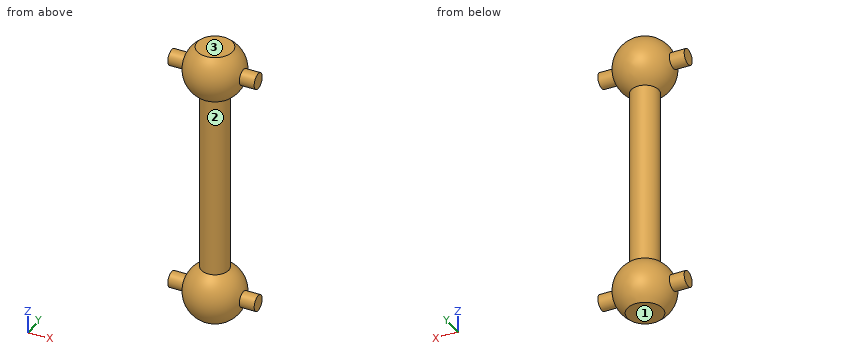
from build123d import *
from build123d.topology import SkipClean

# Parameters (mm, degrees)
SKETCH_1_R      = 3.5
EXTRUDE_1_DEPTH = 25
SKETCH_3_R      = 2
EXTRUDE_2_DEPTH = 11


with BuildPart() as part:
    # Sketch 1 → Extrude 1 (new, symmetric)
    with BuildSketch(Plane.XY):
        Circle(SKETCH_1_R)
    extrude(amount=EXTRUDE_1_DEPTH, both=True)

    # Sketch 2 → Revolve 1 (revolve)
    with SkipClean():  # the faces are left unmerged after this step: merging them gives an invalid solid
        with BuildSketch(Plane(origin=(0, 0, 0), x_dir=(0, 0, -1), z_dir=(1, 0, 0))):
            with BuildLine():
                Line((36, 0), (36, 4.5))
                ThreePointArc((36, 4.5), (27.628291755, 7.115124735), (22.5, 0))
                Line((22.5, 0), (36, 0))
            make_face()
            with BuildLine():
                Line((36, -4.5), (36, 0))
                Line((36, 0), (22.5, 0))
                ThreePointArc((22.5, 0), (27.628291755, -7.115124735), (36, -4.5))
            make_face()
        revolve_1 = revolve(axis=Axis((0, 0, -22.5), (0, 0, -1)))
    add(part.part.scale(1), mode=Mode.REPLACE)  # the faces are merged on a copy

    # Sketch 3 → Extrude 2 (add, symmetric)
    with BuildSketch(Plane(origin=(0, 0, 0), x_dir=(0, 0, -1), z_dir=(1, 0, 0))):
        with Locations(Location((30, 0, 0), (0, 0, 180))):
            Circle(SKETCH_3_R)
    extrude_2 = extrude(amount=EXTRUDE_2_DEPTH, both=True)

    # Mirror 1: Revolve 1, Extrude 2 across plane
    add(revolve_1.mirror(Plane.XY))
    add(extrude_2.mirror(Plane.XY))


solid = part.part
CAD build for the part. Positions are in the model's coordinates, mm. Face numbers are marked on the shaded views. Round coordinates to 2 decimals unless told otherwise and drop trailing zeros. Loops run counter-clockwise (first coordinate to the right, second up) from the corner with the lowest first, then second, coordinate; pieces in that order, holes last.
(1) Cut at B-B (y = 0). Give the cut face in (x, z).
(2) Cut at A-A (x = 0). Give the cut face in (y, z), plus the area to 3 significant figures.
(3) Wall check: line 1 along Y through (x, z) = (-6, -30); line 2 along Z through (x, y) = (-1, -3.5); line 3 along Z through (x, y) = (-5, 1.5). Give the ranges that are in metal, low to high.
(4) Two-plate mould, pull along Z, no slides. Class the marked faces 1, 2 and 3: +Z half, -Z half, draft (parallel to the pull), parting line (faces both ways), or undercut.
(5) Cut at D-D (y = 6.25). Give the cut face in (x, z), plus the area to 3 significant figures.
(6) Cut at C-C (z = -30). Give the cut face in (x, y), plus the area to 3 significant figures.
(7) Drop flat-ended pins along their axis: pin 1 (6 mm diameter, centred on y = -2, z = -15, fed in from +X); pin 2 (1.5 mm diameter, centred on y = 1.5, z = 21.5, fed in from +X); pin 3 (8 mm diameter, centred on y = -5.5, z = -17.5, fed in from +X); pin 4 (6 mm diameter, centred on y = -0.5, z = 27, fed in from -X). Give the stop position or say it passes through.
Findings below:
1. outline: (-11, -32) - (-7.23, -32) arc R7.5 ccw to (-4.5, -36) - (4.5, -36) arc R7.5 ccw to (7.23, -32) - (11, -32) - (11, -28) - (7.23, -28) arc R7.5 ccw to (3.5, -23.37) - (3.5, 23.37) arc R7.5 ccw to (7.23, 28) - (11, 28) - (11, 32) - (7.23, 32) arc R7.5 ccw to (4.5, 36) - (-4.5, 36) arc R7.5 ccw to (-7.23, 32) - (-11, 32) - (-11, 28) - (-7.23, 28) arc R7.5 ccw to (-3.5, 23.37) - (-3.5, -23.37) arc R7.5 ccw to (-7.23, -28) - (-11, -28) - close
2. outline: (-4.5, -36) - (4.5, -36) arc R7.5 ccw to (3.5, -23.37) - (3.5, 23.37) arc R7.5 ccw to (4.5, 36) - (-4.5, 36) arc R7.5 ccw to (-3.5, 23.37) - (-3.5, -23.37) arc R7.5 ccw to start
2. area: 654 mm2
3. line 1: y = -4.5 to 4.5
3. line 2: z = -36 to -23.44, 23.44 to 36
3. line 3: z = -35.39 to -24.61, 24.61 to 35.39
4. face 1: -Z half
4. face 2: undercut
4. face 3: +Z half
5. outline: circle Ø8.29 at (0, -30); circle Ø8.29 at (0, 30)
5. area: 108 mm2
6. outline: (-11, -2) - (-7.23, -2) arc R7.5 ccw to (7.23, -2) - (11, -2) - (11, 2) - (7.23, 2) arc R7.5 ccw to (-7.23, 2) - (-11, 2) - close
6. area: 205 mm2
7. pin 1: stops at x = 3.5
7. pin 2: stops at x = 3.42
7. pin 3: stops at x = 3.16
7. pin 4: stops at x = -11
